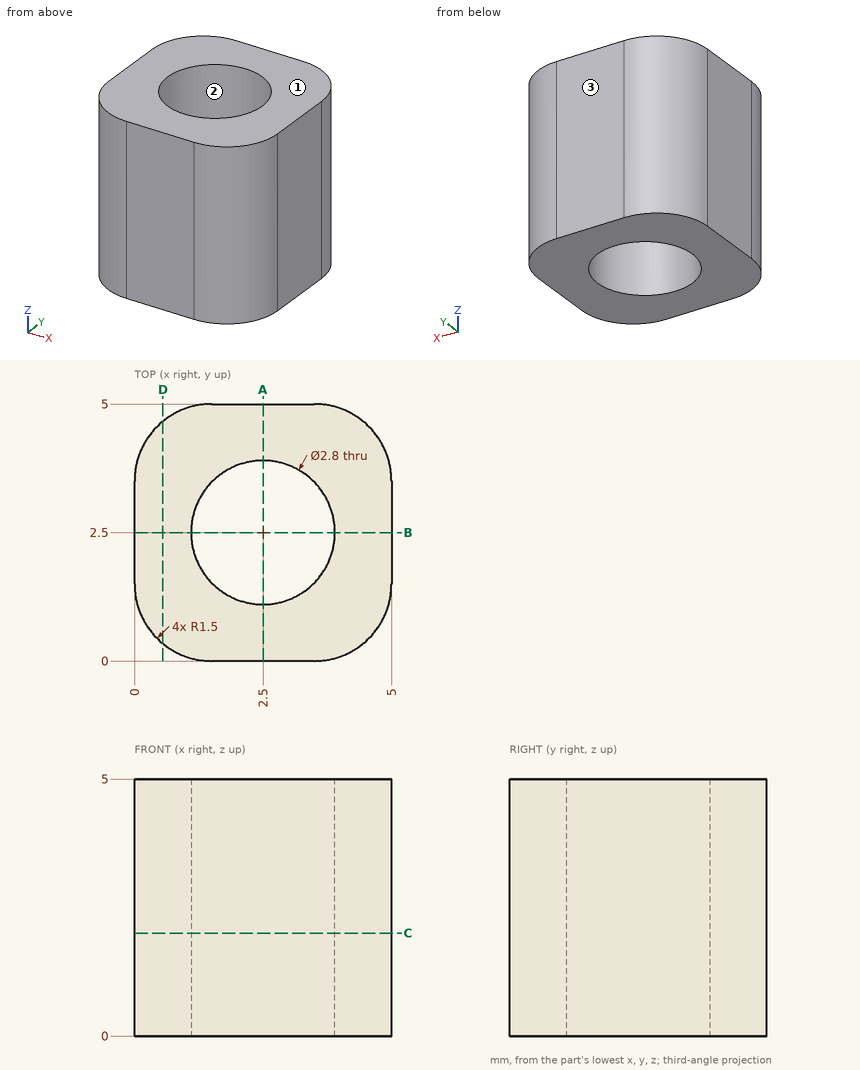
Input: dimensioned drawing with shaded views. Units: mm. Origin: part minimum x, y, z. Round coordinates to 2 decimals unless told otherwise and drop trailing zeros. Order: outer loops, then holes, each group sorted by start corner. A loop starts at its lowest first (then second) coordinate and runs counter-clockwise, first axis right, second up. Notation, with made-up numbers: (73.5, -32.5) -> (124.5, -32.5) arc R23 ccw to (124.5, -22.5) -> close; hole circle Ø4 at (20.5, 54). An arc over 180 degrees is marked (long way). One line per item, written item: value. Start each with the question number.
Q1. Section query D-D (x = 0.55). Return the cut outline in (y, z), plus the area to 3 significant figures.
Q2. Draft query along Y for the marked faces 1, 2 and 3. Return one class per face: pulls with the +Y half, pulls with the -Y half, needs draft (parallel to the pull), parting line crosses it, or undercut.
Q3. Pin query (flat end, axial travel): pin 1 (1.5 mm diameter, centred on y = 1, z = 2, fed in from +X); pin 2 (2.5 mm diameter, centred on x = 2.5, y = 2.5, fed in from -Z). Return the tip coordinate at first contact, or that it passes through.
Q4. Section query C-C (z = 2). Return the cut outline in (x, y).
Q5. Section query A-A (x = 2.5). Return the cut outline in (y, z).
Q6. Material intervals for probe 1 along Y at (x, z) = (2.5, 1); probe 2 along Y at (x, z) = (3.3, 2); probe 3 along X at (y, z) = (2.35, 4.25), sorted ascending.
Findings below:
1. outline: (0.34, 0) -> (4.66, 0) -> (4.66, 5) -> (0.34, 5) -> close
1. area: 21.6 mm²
2. face 1: needs draft
2. face 2: undercut
2. face 3: pulls with the +Y half
3. pin 1: x = 5
3. pin 2: through
4. outline: (0, 1.5) arc R1.5 ccw to (1.5, 0) -> (3.5, 0) arc R1.5 ccw to (5, 1.5) -> (5, 3.5) arc R1.5 ccw to (3.5, 5) -> (1.5, 5) arc R1.5 ccw to (0, 3.5) -> close; hole circle Ø2.8 at (2.5, 2.5)
5. outline: (0, 0) -> (1.1, 0) -> (1.1, 5) -> (0, 5) -> close; (3.9, 0) -> (5, 0) -> (5, 5) -> (3.9, 5) -> close
6. probe 1: 0 to 1.1, 3.9 to 5
6. probe 2: 0 to 1.35, 3.65 to 5
6. probe 3: 0 to 1.11, 3.89 to 5
